from build123d import *

# Parameters (mm, degrees)
F1_DEPTH = 12.7
F3_D     = 3.96875
F4_D     = 12.7
F5_D     = 6.35


with BuildPart() as f1:
    # F0 (on Top) → F1 (new body)
    with BuildSketch(Plane.XY):
        with BuildLine():
            Line((1473.2, -230.5812), (1473.2, 0))
            Line((1473.2, 0), (1473.2, 230.5812))
            ThreePointArc((1473.2, 230.5812), (1458.321024, 266.502224), (1422.4, 281.3812))
            Line((1422.4, 281.3812), (762, 281.3812))
            ThreePointArc((762, 281.3812), (726.078976, 266.502224), (711.2, 230.5812))
            Line((711.2, 230.5812), (711.2, 190.5))
            ThreePointArc((711.2, 190.5), (696.321024, 154.578976), (660.4, 139.7))
            Line((660.4, 139.7), (50.8, 139.7))
            ThreePointArc((50.8, 139.7), (14.878976, 124.821024), (0, 88.9))
            Line((0, 88.9), (0, 0))
            Line((0, 0), (0, -88.9))
            ThreePointArc((0, -88.9), (14.878976, -124.821024), (50.8, -139.7))
            Line((50.8, -139.7), (660.4, -139.7))
            ThreePointArc((660.4, -139.7), (696.321024, -154.578976), (711.2, -190.5))
            Line((711.2, -190.5), (711.2, -230.5812))
            ThreePointArc((711.2, -230.5812), (726.078976, -266.502224), (762, -281.3812))
            Line((762, -281.3812), (1422.4, -281.3812))
            ThreePointArc((1422.4, -281.3812), (1458.321024, -266.502224), (1473.2, -230.5812))
        make_face()
    extrude(amount=F1_DEPTH)

    # F3 (through all)
    with Locations(Plane.XY.offset(12.7)):
        with Locations((749.3, 263.89965), (774.7, 263.89965), (774.7, 221.03715), (749.3, 221.03715), (749.3, -221.03715), (774.7, -221.03715), (774.7, -263.89965), (749.3, -263.89965), (1409.7, -221.03715), (1435.1, -221.03715), (1435.1, -263.89965), (1409.7, -263.89965), (1435.1, 221.03715), (1409.7, 221.03715), (1409.7, 263.89965), (1435.1, 263.89965)):
            Hole(F3_D / 2)

    # F4 (through all)
    with Locations(Plane.XY.offset(12.7)):
        with Locations((965.680041, 101.6), (1218.719959, 101.6), (1218.719959, -101.6), (965.680041, -101.6)):
            Hole(F4_D / 2)

    # F5 (through all)
    with Locations(Plane.XY.offset(12.7)):
        with Locations((25.4, 95.25), (50.8, 95.25), (50.8, -95.25), (25.4, -95.25), (711.2, 95.25), (736.6, 95.25), (736.6, -95.25), (711.2, -95.25)):
            Hole(F5_D / 2)


solid = f1.part
Read the model definition and answer for the solid it produces. Units are mm, in the model's axes. Coordinates: 2 decimals unless noted, no trailing zeros. Write each loop counter-clockwise with the first axis right and the second up, starting at its lowest first coordinate (ties: lowest second). Pieces come first, ordered by that corner, then holes. Notation, with made-up numbers: M 14,77.25 L 38,77.25 A26 cw 38,104.25 Z; hole C -9,-7.75 d10. An arc over 180 degrees is marked long. Use a Markdown table: item, result.
Q1. Each of these flat-tipped pins is pushed along its axis until it touches: pin 1 Ø3 at (x, y) = (1435.1, -263.9) entering from +Z; pin 2 Ø6.5 at (x, z) = (343.5, 8) entering from -Y; pin 3 Ø6.5 at (y, z) = (215.5, 3.5) entering from -X. Where does it stop, or does it pass through?
Answer block:
| item | result |
|---|---|
| pin 1 | passes through |
| pin 2 | stops at y = -139.7 |
| pin 3 | stops at x = 711.2 |
Q2. Straight lines are drawn through the part: L1, parallel to X at y = 221, z = 2.75; L2, parallel to Y at x = 774.7, z = 4.5; L3, parallel to X at y = 106, z = 1.5. For each, find the intervals that lie inside material, in ascending order. Write a range as [from, to].
Answer block:
| item | result |
|---|---|
| L1 | x = [711.2, 747.32], [751.28, 772.72], [776.68, 1407.72], [1411.68, 1433.12], [1437.08, 1473.2] |
| L2 | y = [-281.38, -265.88], [-261.92, -223.02], [-219.05, 219.05], [223.02, 261.92], [265.88, 281.38] |
| L3 | x = [2.96, 961.1], [970.26, 1214.14], [1223.3, 1473.2] |
Q3. The part is cut by section C-C, the plane y = -153.5. Write down the section's boundary in (x, z), then the cut area to 3 significant figures.
Answer block:
| item | result |
|---|---|
| outline | M 695.21,0 L 1473.2,0 L 1473.2,12.7 L 695.21,12.7 Z |
| area | 9,880 mm2 |
Q4. The part is cut by section A-A, the plane x = 163. Write down the section's boundary in (y, z).
Answer block:
| item | result |
|---|---|
| outline | M -139.7,0 L 139.7,0 L 139.7,12.7 L -139.7,12.7 Z |
Q5. The part is cut by section B-B, the plane z = 7.75. Give the number of separate pieces and of enclosed holes in the cut face, then the cut area to 3 significant figures.
Answer block:
| item | result |
|---|---|
| separate pieces | 1 |
| enclosed holes | 28 |
| area | 624,000 mm2 |
